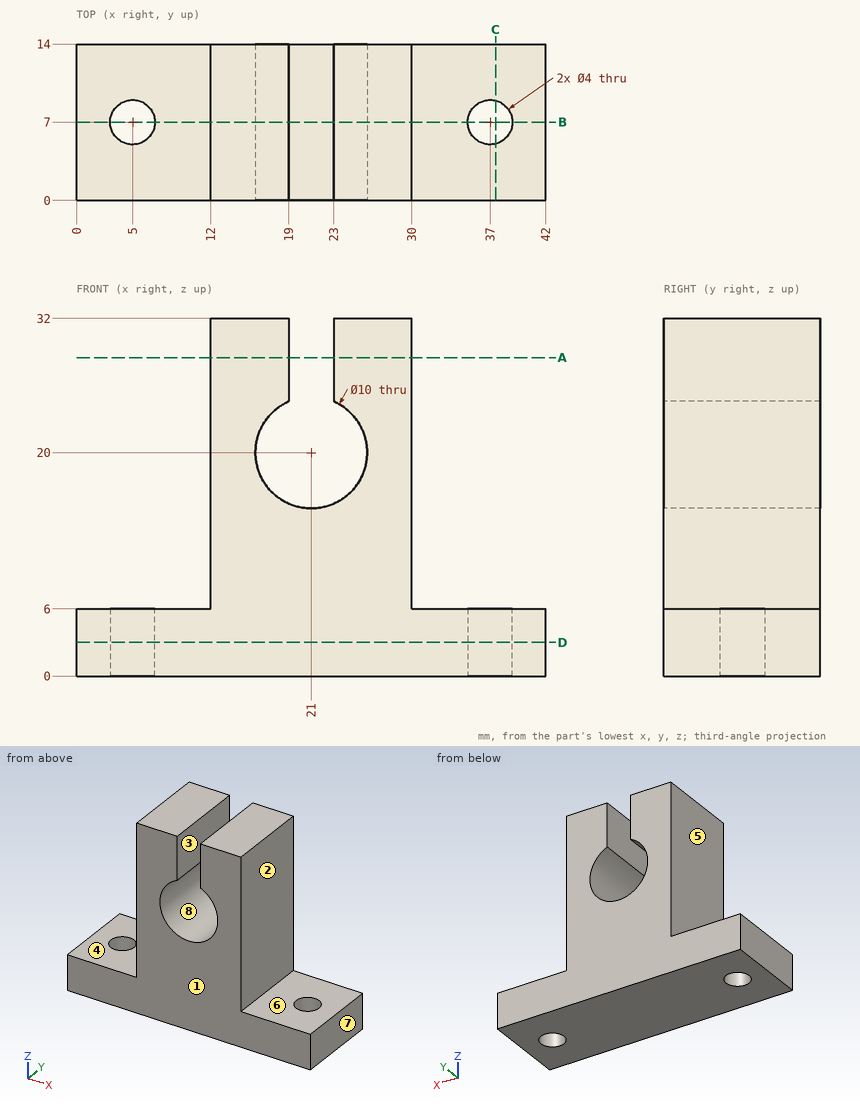
Geometry: see drawing. Coordinates: mm, zero at the bounding-box minimum. A direction names the side the tool comes from. Coordinates: 2 decimals unless noted, no trailing zeros. Loops run counter-clockwise (first coordinate to the right, second up) from the corner with the lowest first, then second, coordinate; pieces in that order, holes last. Notation, with made-up numbers: M -17.75,-0.5 L 28.25,-0.5 A9 ccw 28.25,7.5 Z; hole C 84.5,54 d3. An arc over 180 degrees is marked long. Answer in a Markdown table with one row per item.
1. Section C-C, the plane x = 37.5. Output: boundary loops of the cut face in (y, z).
Response:
| item | result |
|---|---|
| outline | M 0,0 L 5.06,0 L 5.06,6 L 0,6 Z; M 8.94,0 L 14,0 L 14,6 L 8.94,6 Z |
2. Material intervals for line 1 (X direction, y = 7, z = 2.2); line 2 (X direction, y = 6.5, z = 20); line 3 (X direction, y = 12.75, z = 28), sorted ascending.
Response:
| item | result |
|---|---|
| line 1 | x = 0 to 3, 7 to 35, 39 to 42 |
| line 2 | x = 12 to 16, 26 to 30 |
| line 3 | x = 12 to 19, 23 to 30 |
3. Section A-A, the plane z = 28.5. Output: boundary loops of the cut face in (x, y).
Response:
| item | result |
|---|---|
| outline | M 12,0 L 19,0 L 19,14 L 12,14 Z; M 23,0 L 30,0 L 30,14 L 23,14 Z |
4. Section D-D, the plane z = 3. Output: boundary loops of the cut face in (x, y), then the cut area to 3 significant figures.
Response:
| item | result |
|---|---|
| outline | M 0,0 L 42,0 L 42,14 L 0,14 Z; hole C 5,7 d4; hole C 37,7 d4 |
| area | 563 mm2 |
5. Section B-B, the plane y = 7. Output: boundary loops of the cut face in (x, z).
Response:
| item | result |
|---|---|
| outline | M 0,0 L 3,0 L 3,6 L 0,6 Z; M 7,0 L 35,0 L 35,6 L 30,6 L 30,32 L 23,32 L 23,24.58 A5 cw long 19,24.58 L 19,32 L 12,32 L 12,6 L 7,6 Z; M 39,0 L 42,0 L 42,6 L 39,6 Z |
6. Reachability of the marked faces 1, 2, 3 and 4 from +Z, -Z, +X, -X, +Y, -Y: full face, straight path, thin tool, end or side. Return the list, or none.
Response:
| item | result |
|---|---|
| face 1 | +Z, -Z, +X, -X, -Y |
| face 2 | +Z, +X, +Y, -Y |
| face 3 | +Z, +Y, -Y |
| face 4 | +Z, -X, +Y, -Y |
7. Draft query along X for the marked faces 5, 6, 7 and 8. Return one class per face: pulls with the +X half, pulls with the -X half, needs draft (parallel to the pull), parting line crosses it, or undercut.
Response:
| item | result |
|---|---|
| face 5 | pulls with the -X half |
| face 6 | needs draft |
| face 7 | pulls with the +X half |
| face 8 | undercut |
8. First-contact query: pin 1 (8 mm diameter, centred on y = 6.5, z = 30, fed in from -X); pin 2 (6 mm diameter, centred on y = 10, z = 29, fed in from +X). Flat tips, straight axial feed; report the tip coordinate or a pass-through.
Response:
| item | result |
|---|---|
| pin 1 | stops at x = 12 |
| pin 2 | stops at x = 30 |
